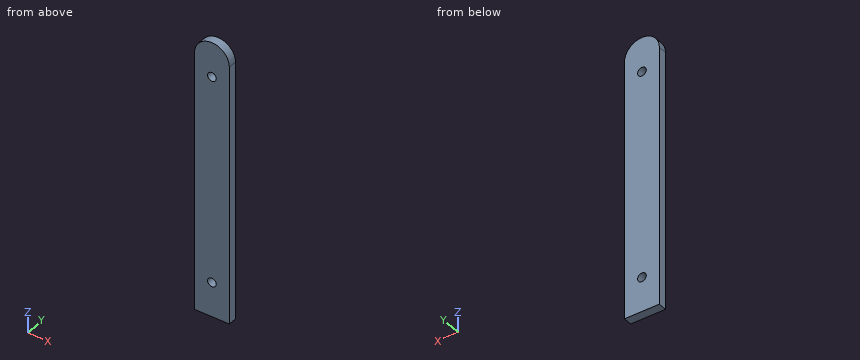
```python
from build123d import *

# Parameters (mm, degrees)
SKETCH1_W           = 25.4
SKETCH1_H           = 203.454
SKETCH1_R           = 3.175
BOSS_EXTRUDE1_DEPTH = 6.35
FILLET1_RADIUS      = 12.7
FILLET1_LENGTH      = 6.35


with BuildPart() as part:
    # Sketch1 → Boss-Extrude1 (new body)
    with BuildSketch(Plane(origin=(0, 0, 0), x_dir=(1, 0, 0), z_dir=(0, 1, 0))):
        with Locations((6.296638655, -73.658932773)):
            Rectangle(SKETCH1_W, SKETCH1_H)
        with Locations(Location((6.296638655, 2.668067227, 0), (0, 0, 270))):
            Circle(SKETCH1_R, mode=Mode.SUBTRACT)
        with Locations(Location((6.296638655, -149.985932773, 0), (0, 0, 270))):
            Circle(SKETCH1_R, mode=Mode.SUBTRACT)
    extrude(amount=BOSS_EXTRUDE1_DEPTH)

    # Fillet1: full round fillet: the end face becomes a half cylinder, R = half its width
    fillet1_face = Plane((6.296638655, 3.175, 175.385932773), x_dir=(0, 1, 0), z_dir=(0, 0, 1))  # on the end face: x along it, z out of the body
    fillet1_slab = fillet1_face.offset(-FILLET1_RADIUS / 2) * Box(FILLET1_LENGTH, 2 * FILLET1_RADIUS, FILLET1_RADIUS, mode=Mode.PRIVATE)  # the body's end, R deep
    fillet1_round = Plane((6.296638655, 3.175, 162.685932773), x_dir=(0, 0, 1), z_dir=(0, 1, 0)) * Cylinder(FILLET1_RADIUS, FILLET1_LENGTH, mode=Mode.PRIVATE)  # its axis R under the face
    add(fillet1_slab - fillet1_round, mode=Mode.SUBTRACT)


solid = part.part
```
For this review, take the finished solid that the model builds, in its own axes (mm). Round coordinates to 2 decimals unless told otherwise and drop trailing zeros. Write each loop counter-clockwise with the first axis right and the second up, starting at its lowest first coordinate (ties: lowest second). Pieces come first, ordered by that corner, then holes. Notation, with made-up numbers: (63.5, 89) - (72.5, 89) arc R19 cw to (72.5, 103) - close; hole circle Ø5 at (78.25, 85.5). An arc over 180 degrees is marked (long way). Write each question's results on one line, items separated by ' | '.
Item 1: For pin 1 (5 mm diameter, centred on x = 14.5, z = 119.5, fed in from -Y); pin 2 (5.5 mm diameter, centred on x = 6.3, z = 149.99, fed in from -Y) (1 decimal); pin 3 (3 mm diameter, centred on x = 1.5, y = 4.5, fed in from +Z), all flat-tipped, find the tip position at first contact; note any pin that passes through.
Calculated:
pin 1: stops at y = 0 | pin 2: passes through | pin 3: stops at z = 174.95
Item 2: Take a section at C-C on x = 17. State the section outline as (y, z) points.
Calculated:
outline: (0, -28.07) - (6.35, -28.07) - (6.35, 169.52) - (0, 169.52) - close
Item 3: To check wall thickness, follow line 1 along Z through (x, y) = (8.5, 3.75); line 2 along Z through (x, y) = (7, 3); line 3 along X through (y, z) = (5.5, -4). State the ranges of each line that lie inside material, in increasing order. Write a range as from..to.
Calculated:
line 1: z = -28.07..-4.95, -0.38..147.7, 152.27..175.19 | line 2: z = -28.07..-5.76, 0.43..146.89, 153.08..175.37 | line 3: x = -6.4..3.41, 9.18..19
Item 4: Take a section at A-A on y = 4.5. State the section outline as (x, z) points (3 decimals), then the cut area to 3 significant figures.
Calculated:
outline: (-6.403, -28.068) - (18.997, -28.068) - (18.997, 162.686) arc R12.7 ccw to (-6.403, 162.686) - close; hole circle Ø6.35 at (6.297, -2.668); hole circle Ø6.35 at (6.297, 149.986) | area: 5,040 mm^2
Item 5: Take a section at B-B on x = -2.5. State the section outline as (y, z) points, then the cut area to 3 significant figures.
Calculated:
outline: (0, -28.07) - (6.35, -28.07) - (6.35, 171.85) - (0, 171.85) - close | area: 1,270 mm^2
